Can you work these out from the model? Positions are in its coordinate system, mm. A direction names the side the tool comes from. Round coordinates to 2 decimals unless told otherwise and drop trailing zeros. Loops run counter-clockwise (first coordinate to the right, second up) from the corner with the lowest first, then second, coordinate; pieces in that order, holes last. Notation, with made-up numbers: M 57.5,24.5 L 64.5,24.5 A19 ccw 64.5,61.5 Z; hole C 31,-25 d1. An arc over 180 degrees is marked long. Answer as CSV lines item,"result".
from build123d import *

# Parameters (mm, degrees)
SKETCH_2_W          = 40
SKETCH_2_H          = 39
EXTRUDE_1_DEPTH     = 20
FILLET_1_R          = 1
SKETCH_7_W          = 18
SKETCH_7_H          = 2
EXTRUDE_3_DEPTH     = 7
SKETCH_8_W          = 18
SKETCH_8_H          = 2
EXTRUDE_4_DEPTH     = 7
SKETCH_11_R         = 1
CUT_EXTRUDE_2_DEPTH = 62.079339492
SKETCH_12_R         = 4.5
EXTRUDE_5_DEPTH     = 2
SKETCH_13_R         = 1.5
EXTRUDE_6_DEPTH     = 4
FILLET_2_R          = 0.5
FILLET_3_R          = 0.5
FILLET_4_R          = 0.5
SKETCH_10_R         = 1
CUT_EXTRUDE_3_DEPTH = 62.079339492


with BuildPart() as part:
    # 草图2 → 凸台-拉伸1 (new body)
    with BuildSketch(Plane.XY):
        with Locations((-21.679417753, 9.546852913)):
            Rectangle(SKETCH_2_W, SKETCH_2_H)
    extrude(amount=EXTRUDE_1_DEPTH)

    # 圆角1
    fillet_1_edges = [part.edges().sort_by_distance(p)[0] for p in [
        (-1.679417753, 9.546852913, 20),
        (-21.679417753, 29.046852913, 20),
        (-41.679417753, 9.546852913, 20),
        (-21.679417753, 29.046852913, 0),
        (-1.679417753, 9.546852913, 0),
        (-21.679417753, -9.953147087, 0),
        (-41.679417753, 9.546852913, 0),
        (-41.679417753, 29.046852913, 10),
        (-1.679417753, 29.046852913, 10),
        (-1.679417753, -9.953147087, 10),
        (-41.679417753, -9.953147087, 10),
        (-21.679417753, -9.953147087, 20),
    ]]
    fillet(fillet_1_edges, radius=FILLET_1_R)

    # 草图7 → 凸台-拉伸3 (add)
    with BuildSketch(Plane.ZY.offset(41.679417753)):
        with Locations((10, 20.046852913)):
            Rectangle(SKETCH_7_W, SKETCH_7_H)
    extrude(amount=EXTRUDE_3_DEPTH)

    # 草图8 → 凸台-拉伸4 (add)
    with BuildSketch(Plane(origin=(-1.679417753, 0, 0), x_dir=(0, 0, -1), z_dir=(1, 0, 0))):
        with Locations((-10, 20.046852913)):
            Rectangle(SKETCH_8_W, SKETCH_8_H)
    extrude(amount=EXTRUDE_4_DEPTH)

    # 草图11 → 切除-拉伸2 (cut, through all)
    with BuildSketch(Plane(origin=(0, 21.046852913, 0), x_dir=(1, 0, 0), z_dir=(0, 1, 0))):
        with Locations(Location((2.320582247, -5, 0), (0, 0, 270))):
            Circle(SKETCH_11_R)
        with Locations(Location((2.320582247, -15, 0), (0, 0, 270))):
            Circle(SKETCH_11_R)
    extrude(amount=-CUT_EXTRUDE_2_DEPTH, mode=Mode.SUBTRACT)

    # 草图12 → 凸台-拉伸5 (add)
    with BuildSketch(Plane(origin=(0, 29.046852913, 0), x_dir=(1, 0, 0), z_dir=(0, 1, 0))):
        with Locations(Location((-31.679417753, -10, 0), (0, 0, 270))):
            Circle(SKETCH_12_R)
    extrude(amount=EXTRUDE_5_DEPTH)

    # 草图13 → 凸台-拉伸6 (add)
    with BuildSketch(Plane(origin=(0, 29.046852913, 0), x_dir=(1, 0, 0), z_dir=(0, 1, 0))):
        with Locations(Location((-31.679417753, -10, 0), (0, 0, 270))):
            Circle(SKETCH_13_R)
    extrude(amount=EXTRUDE_6_DEPTH)

    # 圆角2
    fillet_2_edges = [part.edges().sort_by_distance(p)[0] for p in [
        (-31.679417753, 31.046852913, 5.5),
    ]]
    fillet(fillet_2_edges, radius=FILLET_2_R)

    # 草图17 → M3 螺纹孔的螺纹孔钻头1 (revolve, cut)
    with BuildSketch(Plane(origin=(-31.679417753, 33.046852913, 10), x_dir=(0, 0, 1), z_dir=(1, 0, 0))):
        Polygon((0, 0), (0, 0.801075774), (1.25, 0.05), (1.25, 0.025), (1.275, 0), align=None)
    revolve(axis=Axis((-31.679417753, 39.396852913, 10), (0, -1, 0)), mode=Mode.SUBTRACT)

    # 圆角3
    fillet_3_edges = [part.edges().sort_by_distance(p)[0] for p in [
        (-48.679417753, 20.046852913, 1),
        (-45.179417753, 21.046852913, 1),
        (-48.679417753, 19.046852913, 10),
        (-45.179417753, 19.046852913, 1),
        (-48.679417753, 20.046852913, 19),
        (-45.179417753, 19.046852913, 19),
        (-48.679417753, 21.046852913, 10),
        (-45.179417753, 21.046852913, 19),
    ]]
    fillet(fillet_3_edges, radius=FILLET_3_R)

    # 圆角4
    fillet_4_edges = [part.edges().sort_by_distance(p)[0] for p in [
        (1.820582247, 21.046852913, 19),
        (1.820582247, 19.046852913, 19),
        (1.820582247, 19.046852913, 1),
        (1.820582247, 21.046852913, 1),
        (5.320582247, 20.046852913, 19),
        (5.320582247, 19.046852913, 10),
        (5.320582247, 20.046852913, 1),
        (5.320582247, 21.046852913, 10),
    ]]
    fillet(fillet_4_edges, radius=FILLET_4_R)

    # 草图10 → 切除-拉伸3 (cut, through all)
    with BuildSketch(Plane(origin=(0, 21.046852913, 0), x_dir=(1, 0, 0), z_dir=(0, 1, 0))):
        with Locations(Location((-45.679417753, -5, 0), (0, 0, 270))):
            Circle(SKETCH_10_R)
        with Locations(Location((-45.679417753, -15, 0), (0, 0, 270))):
            Circle(SKETCH_10_R)
    extrude(amount=-CUT_EXTRUDE_3_DEPTH, mode=Mode.SUBTRACT)


solid = part.part
Item 1: We'd pull the mould along Z, two halves only. Please class faces 5 (the face through (-44.84, 20.06, 15.54)), 6 (the face through (-22, 10, 20)), 7 (the face through (-41.679, 5, 10)): released by +Z, released by -Z, zero draft, split by the parting line, or undercut.
Output:
face 5,"undercut"
face 6,"released by +Z"
face 7,"zero draft"
Item 2: If we section it at B-B on x = -14.5: Write out the boundary of the cut face in (y, z), then the cut area to 3 significant figures.
Output:
outline,"M -9.95,1 A1 ccw -8.95,0 L 28.05,0 A1 ccw 29.05,1 L 29.05,19 A1 ccw 28.05,20 L -8.95,20 A1 ccw -9.95,19 Z"
area,"779 mm2"
Item 3: If we section it at A-A on z = 3: Write out the boundary of the cut face in (x, y).
Output:
outline,"M -48.68,19.55 A0.5 ccw -48.18,19.05 L -41.68,19.05 L -41.68,-8.95 A1 ccw -40.68,-9.95 L -2.68,-9.95 A1 ccw -1.68,-8.95 L -1.68,19.05 L 4.82,19.05 A0.5 ccw 5.32,19.55 L 5.32,20.55 A0.5 ccw 4.82,21.05 L -1.68,21.05 L -1.68,28.05 A1 ccw -2.68,29.05 L -40.68,29.05 A1 ccw -41.68,28.05 L -41.68,21.05 L -48.18,21.05 A0.5 ccw -48.68,20.55 Z"
Item 4: Will these pins go through, and if not, where does the flat tip stop? pin 1 (2 mm diameter, centred on x = -43.5, z = 7, fed in from -Y); pin 2 (5.5 mm diameter, centred on x = -24.5, z = 13, fed in from +Y); pin 3 (1.5 mm diameter, centred on y = 25, z = 2, fed in from -X).
Output:
pin 1,"stops at y = 19.05"
pin 2,"stops at y = 29.05"
pin 3,"stops at x = -41.68"
Item 5: On a 3-axis mill with a long thin cutter (end or side, diameter ignored), from which of +Z, -Z, +X, -X, +Y, -Y can I reach the whole of each face in a straight line? I mean faces 1 (the face through (-1.679, 5, 10)), 2 (the face through (-30.328, 29.786, 14.292)), 3 (the face through (-45, 19.047, 10)), 4 (the face through (2, 21.047, 10)). Say none if no direction works.
Output:
face 1,"+Z, -Z, +X, -Y"
face 2,"+Y"
face 3,"+Z, -Z, -X, -Y"
face 4,"+Z, -Z, +X, +Y"
Item 6: If I drill on line 1 along X through (y, z) = (19.95, 5); line 2 along X through (y, z) = (33, 10); line 3 along X through (y, z) = (4, 1.5), over which ranges is the centre line in solid material (lowest first)? Write a range as from..to.
Output:
line 1,"x = -48.68..-46.68, -44.68..1.32, 3.32..5.32"
line 2,"x = -33.18..-32.93, -30.43..-30.18"
line 3,"x = -41.68..-1.68"
Item 7: If we section it at C-C on y = 4: Write out the boundary of the cut face in (x, z).
Output:
outline,"M -41.68,1 A1 ccw -40.68,0 L -2.68,0 A1 ccw -1.68,1 L -1.68,19 A1 ccw -2.68,20 L -40.68,20 A1 ccw -41.68,19 Z"
